The model under review builds one solid part; all positions refer to its coordinate system, in mm. A direction names the side the tool comes from. Round coordinates to 2 decimals unless told otherwise and drop trailing zeros. Order: outer loops, then holes, each group sorted by start corner. A loop starts at its lowest first (then second) coordinate and runs counter-clockwise, first axis right, second up. Notation, with made-up numbers: (68, 13.5) -> (88, 13.5) arc R19 ccw to (88, 41.5) -> close; hole circle Ø1 at (62.25, -36.5). An arc over 180 degrees is marked (long way). Use a Markdown table: item, result. Add a question column.
```python
from build123d import *

# Parameters (mm, degrees)
SKETCH_1_W          = 36
SKETCH_1_H          = 36
EXTRUDE_1_DEPTH     = 12
SKETCH_2_W          = 25
SKETCH_2_H          = 25
EXTRUDE_2_DEPTH     = 2
SKETCH_3_R          = 7
EXTRUDE_3_DEPTH     = 10
FILLET_1_R          = 2
FILLET_2_R          = 1
FILLET_3_R          = 1
SKETCH_4_R          = 1
CUT_EXTRUDE_1_DEPTH = 50


with BuildPart() as part:
    # 草图1 → 凸台-拉伸1 (new body)
    with BuildSketch(Plane(origin=(0, 0, 0), x_dir=(1, 0, 0), z_dir=(0, 1, 0))):
        Rectangle(SKETCH_1_W, SKETCH_1_H)
    extrude(amount=EXTRUDE_1_DEPTH)

    # 草图2 → 凸台-拉伸2 (add)
    with BuildSketch(Plane(origin=(0, 12, 0), x_dir=(1, 0, 0), z_dir=(0, 1, 0))):
        Rectangle(SKETCH_2_W, SKETCH_2_H)
    extrude(amount=EXTRUDE_2_DEPTH)

    # 草图3 → 凸台-拉伸3 (add)
    with BuildSketch(Plane(origin=(0, 14, 0), x_dir=(1, 0, 0), z_dir=(0, 1, 0))):
        with Locations(Location((0, 0, 0), (0, 0, 270))):
            Circle(SKETCH_3_R)
    extrude(amount=EXTRUDE_3_DEPTH)

    # 圆角1
    fillet_1_edges = [part.edges().sort_by_distance(p)[0] for p in [
        (0, 24, -7),
    ]]
    fillet(fillet_1_edges, radius=FILLET_1_R)

    # 圆角2
    fillet_2_edges = [part.edges().sort_by_distance(p)[0] for p in [
        (0, 12, -12.5),
        (12.5, 12, 0),
        (0, 12, 12.5),
        (-12.5, 14, 0),
        (-12.5, 12, 0),
        (0, 14, 12.5),
        (12.5, 14, 0),
        (0, 14, -12.5),
    ]]
    fillet(fillet_2_edges, radius=FILLET_2_R - 0.0001)  # a hair under: the kernel refuses the full size

    # 圆角3
    fillet_3_edges = [part.edges().sort_by_distance(p)[0] for p in [
        (-18, 12, 0),
        (0, 12, 18),
        (18, 12, 0),
        (0, 0, 18),
        (-18, 0, 0),
        (0, 0, -18),
        (18, 0, 0),
        (18, 6, 18),
        (-18, 6, 18),
        (-18, 6, -18),
        (18, 6, -18),
        (0, 12, -18),
    ]]
    fillet(fillet_3_edges, radius=FILLET_3_R)

    # 草图4 → 切除-拉伸1 (cut)
    with BuildSketch(Plane(origin=(18, 0, 0), x_dir=(0, 0, -1), z_dir=(1, 0, 0))):
        with Locations((0, 6)):
            Circle(SKETCH_4_R)
    extrude(amount=-CUT_EXTRUDE_1_DEPTH, mode=Mode.SUBTRACT)


solid = part.part
```
Q1. For pin 1 (8 mm diameter, centred on x = 4.5, z = -4.5, fed in from +Y); pin 2 (6 mm diameter, centred on x = -6.5, y = 21, fed in from +Z), all flat-tipped, find the tip position at first contact; note any pin that passes through.
Q2. Add section A-A, the plane y = 6. Give the boundary of the cut face in (x, z).
Q3. For faces 5 (the face through (-17.715, 6.07, -17.699)), 6 (the face through (-15, 12, 0)), list the 3-axis set-ups (+Z, -Z, +X, -X, +Y, -Y) from which the entire face can be reached by the end or side of a thin tool; tool diameter is ignored.
Q4. Draft analysis for pull direction Z (two halves, no side actions). For faces 1 (the face through (0, 7, 0)), 2 (the face through (-6.834, 17.944, -1.517)), 3 (the face through (-12.785, 12.301, -0.189)), 4 (the face through (0.175, 13.715, -12.199)), state which applies: released by +Z, released by -Z, zero draft, split by the parting line, or undercut.
Q5. To check wall thickness, follow line 1 along Y through (x, z) = (8, 0); line 2 along Y through (x, z) = (2, 0); line 3 along Y through (x, z) = (-6, -6). State the ranges of each line that lie inside material, in increasing order.
Q6. Add section D-D, the plane z = 16. Give the boundary of the cut face in (x, y), then the cut area to 3 significant figures.
Return value:
| question | item | result |
|---|---|---|
| 1 | pin 1 | y = 24 |
| 1 | pin 2 | z = 6.06 |
| 2 | outline | (-18, -17) arc R1 ccw to (-17, -18) -> (17, -18) arc R1 ccw to (18, -17) -> (18, -1) -> (-18, -1) -> close; (-18, 1) -> (18, 1) -> (18, 17) arc R1 ccw to (17, 18) -> (-17, 18) arc R1 ccw to (-18, 17) -> close |
| 3 | face 5 | -Z, -X, +Y, -Y |
| 3 | face 6 | +Y |
| 4 | face 1 | undercut |
| 4 | face 2 | split by the parting line |
| 4 | face 3 | zero draft |
| 4 | face 4 | released by -Z |
| 5 | line 1 | 0 to 5, 7 to 14 |
| 5 | line 2 | 0 to 5, 7 to 24 |
| 5 | line 3 | 0 to 14 |
| 6 | outline | (-18, 1) arc R1 ccw to (-17, 0) -> (17, 0) arc R1 ccw to (18, 1) -> (18, 11) arc R1 ccw to (17, 12) -> (-17, 12) arc R1 ccw to (-18, 11) -> close |
| 6 | area | 431 mm² |
